from build123d import *

# Parameters (mm, degrees)
SM_BASE_FLANGE_1_DEPTH           = 3
SM_EDGE_FLANGE_1_STRIP_W         = 18
SM_EDGE_FLANGE_1_STRIP_H         = 3
SM_EDGE_FLANGE_1_STRIP_CUT_DEPTH = 130
SM_EDGE_FLANGE_1_DEPTH           = 130
SM_EDGE_FLANGE_2_DEPTH           = 52
SM_EDGE_FLANGE_5_DEPTH           = 52
CUT_EXTRUDE_2_REACH              = 158.911
SKETCH_48_R                      = 3.5
CUT_EXTRUDE_3_REACH              = 150.997
SKETCH_49_R                      = 3.5
CUT_EXTRUDE_4_REACH              = 150.997
SKETCH_51_R                      = 3.5
SM_EDGE_FLANGE_6_DEPTH           = 52
CUT_EXTRUDE_5_REACH              = 263.117
SKETCH_59_R                      = 3.5
SM_EDGE_FLANGE_8_DEPTH           = 130
CUT_EXTRUDE_6_REACH              = 229.141
SKETCH_68_R                      = 3.5
CUT_EXTRUDE_7_REACH              = 198.876
SKETCH_69_R                      = 3.5


# Sheet-metal steps are written as plain solids
with BuildPart() as part:
    # Sketch 2 → Базовая кромка1 (new body)
    with BuildSketch(Plane(origin=(0, 0, 0), x_dir=(1, 0, 0), z_dir=(0, 1, 0))):
        Polygon((45, 55), (130, 55), (130, 35), (45, 0), (0, 0), (0, 55), align=None)
    extrude(amount=-SM_BASE_FLANGE_1_DEPTH)

    # Ребро-кромка1 strip (across the edge) → Ребро-кромка1 strip cut (cut)
    with BuildSketch(Plane(origin=(0, -3, -55), x_dir=(0, 0, 1), z_dir=(1, 0, 0))):
        with Locations((-6, -1.5)):
            Rectangle(SM_EDGE_FLANGE_1_STRIP_W, SM_EDGE_FLANGE_1_STRIP_H)
    extrude(amount=SM_EDGE_FLANGE_1_STRIP_CUT_DEPTH, mode=Mode.SUBTRACT)

    # Ребро-кромка1 section (across the edge) → Ребро-кромка1 (add)
    with BuildSketch(Plane(origin=(0, -3, -55), x_dir=(0, 0, 1), z_dir=(1, 0, 0))):
        with BuildLine():
            Line((-3, 3), (-3, 20))
            Line((-3, 20), (0, 20))
            Line((0, 20), (0, 3))
            ThreePointArc((0, 3), (0.878679656, 0.878679656), (3, 0))
            Line((3, 0), (3, -3))
            ThreePointArc((3, -3), (-1.242640687, -1.242640687), (-3, 3))
        make_face()
    extrude(amount=SM_EDGE_FLANGE_1_DEPTH)

    # Ребро-кромка2 section (across the edge) → Ребро-кромка2 (add)
    with BuildSketch(Plane(origin=(-6, -3, 0), x_dir=(1, 0, 0), z_dir=(0, 0, -1))):
        with BuildLine():
            Line((-3, 3), (-3, 35))
            Line((-3, 35), (0, 35))
            Line((0, 35), (0, 3))
            ThreePointArc((0, 3), (0.878679656, 0.878679656), (3, 0))
            Line((3, 0), (6, 0))
            Line((6, 0), (6, -3))
            Line((6, -3), (3, -3))
            ThreePointArc((3, -3), (-1.242640687, -1.242640687), (-3, 3))
        make_face()
    extrude(amount=SM_EDGE_FLANGE_2_DEPTH)

    # Ребро-кромка5 section (across the edge) → Ребро-кромка5 (add)
    with BuildSketch(Plane(origin=(-9, -41, -52), x_dir=(0, 1, 0), z_dir=(0, 0, 1))):
        with BuildLine():
            Line((-3, 3), (-3, 38))
            Line((-3, 38), (0, 38))
            Line((0, 38), (0, 3))
            ThreePointArc((0, 3), (0.878679656, 0.878679656), (3, 0))
            Line((3, 0), (3, -3))
            ThreePointArc((3, -3), (-1.242640687, -1.242640687), (-3, 3))
        make_face()
    extrude(amount=SM_EDGE_FLANGE_5_DEPTH)

    # Эскиз48 → Вырез-Вытянуть2 (cut, up to next)
    with BuildSketch(Plane.ZY.offset(9), mode=Mode.PRIVATE) as cut_extrude_2_sk1:
        with Locations(Location((-41, -24, 0), (0, 0, 270))):
            Circle(SKETCH_48_R)
    cut_extrude_2_tool1 = extrude(cut_extrude_2_sk1.sketch, amount=-CUT_EXTRUDE_2_REACH, mode=Mode.PRIVATE) & part.part
    # Эскиз48 → Вырез-Вытянуть2 (cut, up to next)
    with BuildSketch(Plane.ZY.offset(9), mode=Mode.PRIVATE) as cut_extrude_2_sk2:
        with Locations(Location((-11, -24, 0), (0, 0, 270))):
            Circle(SKETCH_48_R)
    cut_extrude_2_tool2 = extrude(cut_extrude_2_sk2.sketch, amount=-CUT_EXTRUDE_2_REACH, mode=Mode.PRIVATE) & part.part
    add(cut_extrude_2_tool1.solids().sort_by_distance((-9, -24, -41))[0], mode=Mode.SUBTRACT)
    add(cut_extrude_2_tool2.solids().sort_by_distance((-9, -24, -11))[0], mode=Mode.SUBTRACT)

    # Эскиз49 → Вырез-Вытянуть3 (cut, up to next)
    with BuildSketch(Plane(origin=(0, 0, 0), x_dir=(1, 0, 0), z_dir=(0, 1, 0)), mode=Mode.PRIVATE) as cut_extrude_3_sk1:
        with Locations(Location((21, 12.448418776, 0), (0, 0, 270))):
            Circle(SKETCH_49_R)
    cut_extrude_3_tool1 = extrude(cut_extrude_3_sk1.sketch, amount=-CUT_EXTRUDE_3_REACH, mode=Mode.PRIVATE) & part.part
    # Эскиз49 → Вырез-Вытянуть3 (cut, up to next)
    with BuildSketch(Plane(origin=(0, 0, 0), x_dir=(1, 0, 0), z_dir=(0, 1, 0)), mode=Mode.PRIVATE) as cut_extrude_3_sk2:
        with Locations(Location((21, 38.45, 0), (0, 0, 270))):
            Circle(SKETCH_49_R)
    cut_extrude_3_tool2 = extrude(cut_extrude_3_sk2.sketch, amount=-CUT_EXTRUDE_3_REACH, mode=Mode.PRIVATE) & part.part
    # Эскиз49 → Вырез-Вытянуть3 (cut, up to next)
    with BuildSketch(Plane(origin=(0, 0, 0), x_dir=(1, 0, 0), z_dir=(0, 1, 0)), mode=Mode.PRIVATE) as cut_extrude_3_sk3:
        with Locations(Location((117, 38.45, 0), (0, 0, 270))):
            Circle(SKETCH_49_R)
    cut_extrude_3_tool3 = extrude(cut_extrude_3_sk3.sketch, amount=-CUT_EXTRUDE_3_REACH, mode=Mode.PRIVATE) & part.part
    # Эскиз49 → Вырез-Вытянуть3 (cut, up to next)
    with BuildSketch(Plane(origin=(0, 0, 0), x_dir=(1, 0, 0), z_dir=(0, 1, 0)), mode=Mode.PRIVATE) as cut_extrude_3_sk4:
        with Locations(Location((69, 38.45, 0), (0, 0, 270))):
            Circle(SKETCH_49_R)
    cut_extrude_3_tool4 = extrude(cut_extrude_3_sk4.sketch, amount=-CUT_EXTRUDE_3_REACH, mode=Mode.PRIVATE) & part.part
    add(cut_extrude_3_tool1.solids().sort_by_distance((21, 0, -12.448419))[0], mode=Mode.SUBTRACT)
    add(cut_extrude_3_tool2.solids().sort_by_distance((21, 0, -38.45))[0], mode=Mode.SUBTRACT)
    add(cut_extrude_3_tool3.solids().sort_by_distance((117, 0, -38.45))[0], mode=Mode.SUBTRACT)
    add(cut_extrude_3_tool4.solids().sort_by_distance((69, 0, -38.45))[0], mode=Mode.SUBTRACT)

    # Эскиз51 → Вырез-Вытянуть4 (cut, up to next)
    with BuildSketch(Plane(origin=(0, 0, -58), x_dir=(-1, 0, 0), z_dir=(0, 0, -1)), mode=Mode.PRIVATE) as cut_extrude_4_sk1:
        with Locations(Location((-117, -14.5, 0), (0, 0, 90))):
            Circle(SKETCH_51_R)
    cut_extrude_4_tool1 = extrude(cut_extrude_4_sk1.sketch, amount=-CUT_EXTRUDE_4_REACH, mode=Mode.PRIVATE) & part.part
    # Эскиз51 → Вырез-Вытянуть4 (cut, up to next)
    with BuildSketch(Plane(origin=(0, 0, -58), x_dir=(-1, 0, 0), z_dir=(0, 0, -1)), mode=Mode.PRIVATE) as cut_extrude_4_sk2:
        with Locations(Location((-69, -14.5, 0), (0, 0, 90))):
            Circle(SKETCH_51_R)
    cut_extrude_4_tool2 = extrude(cut_extrude_4_sk2.sketch, amount=-CUT_EXTRUDE_4_REACH, mode=Mode.PRIVATE) & part.part
    # Эскиз51 → Вырез-Вытянуть4 (cut, up to next)
    with BuildSketch(Plane(origin=(0, 0, -58), x_dir=(-1, 0, 0), z_dir=(0, 0, -1)), mode=Mode.PRIVATE) as cut_extrude_4_sk3:
        with Locations(Location((-21, -14.5, 0), (0, 0, 90))):
            Circle(SKETCH_51_R)
    cut_extrude_4_tool3 = extrude(cut_extrude_4_sk3.sketch, amount=-CUT_EXTRUDE_4_REACH, mode=Mode.PRIVATE) & part.part
    add(cut_extrude_4_tool1.solids().sort_by_distance((117, -14.5, -58))[0], mode=Mode.SUBTRACT)
    add(cut_extrude_4_tool2.solids().sort_by_distance((69, -14.5, -58))[0], mode=Mode.SUBTRACT)
    add(cut_extrude_4_tool3.solids().sort_by_distance((21, -14.5, -58))[0], mode=Mode.SUBTRACT)

    # Ребро-кромка6 section (across the edge) → Ребро-кромка6 (add)
    with BuildSketch(Plane(origin=(-50, -44, 0), x_dir=(1, 0, 0), z_dir=(0, 0, -1))):
        with BuildLine():
            Line((-3, 3), (-3, 133))
            Line((-3, 133), (0, 133))
            Line((0, 133), (0, 3))
            ThreePointArc((0, 3), (0.878679656, 0.878679656), (3, 0))
            Line((3, 0), (3, -3))
            ThreePointArc((3, -3), (-1.242640687, -1.242640687), (-3, 3))
        make_face()
    extrude(amount=SM_EDGE_FLANGE_6_DEPTH)

    # Эскиз59 → Вырез-Вытянуть5 (cut, up to next)
    with BuildSketch(Plane.ZY.offset(53), mode=Mode.PRIVATE) as cut_extrude_5_sk1:
        with Locations(Location((-7.981818004, -68, 0), (0, 0, 270))):
            Circle(SKETCH_59_R)
    cut_extrude_5_tool1 = extrude(cut_extrude_5_sk1.sketch, amount=-CUT_EXTRUDE_5_REACH, mode=Mode.PRIVATE) & part.part
    # Эскиз59 → Вырез-Вытянуть5 (cut, up to next)
    with BuildSketch(Plane.ZY.offset(53), mode=Mode.PRIVATE) as cut_extrude_5_sk2:
        with Locations(Location((-37.994919226, -68, 0), (0, 0, 270))):
            Circle(SKETCH_59_R)
    cut_extrude_5_tool2 = extrude(cut_extrude_5_sk2.sketch, amount=-CUT_EXTRUDE_5_REACH, mode=Mode.PRIVATE) & part.part
    # Эскиз59 → Вырез-Вытянуть5 (cut, up to next)
    with BuildSketch(Plane.ZY.offset(53), mode=Mode.PRIVATE) as cut_extrude_5_sk3:
        with Locations(Location((-37.994919226, -116, 0), (0, 0, 270))):
            Circle(SKETCH_59_R)
    cut_extrude_5_tool3 = extrude(cut_extrude_5_sk3.sketch, amount=-CUT_EXTRUDE_5_REACH, mode=Mode.PRIVATE) & part.part
    # Эскиз59 → Вырез-Вытянуть5 (cut, up to next)
    with BuildSketch(Plane.ZY.offset(53), mode=Mode.PRIVATE) as cut_extrude_5_sk4:
        with Locations(Location((-37.994919226, -164, 0), (0, 0, 270))):
            Circle(SKETCH_59_R)
    cut_extrude_5_tool4 = extrude(cut_extrude_5_sk4.sketch, amount=-CUT_EXTRUDE_5_REACH, mode=Mode.PRIVATE) & part.part
    # Эскиз59 → Вырез-Вытянуть5 (cut, up to next)
    with BuildSketch(Plane.ZY.offset(53), mode=Mode.PRIVATE) as cut_extrude_5_sk5:
        Polygon((0, -92), (-35, -177), (0, -177), align=None)
    cut_extrude_5_tool5 = extrude(cut_extrude_5_sk5.sketch, amount=-CUT_EXTRUDE_5_REACH, mode=Mode.PRIVATE) & part.part
    add(cut_extrude_5_tool1.solids().sort_by_distance((-53, -68, -7.981818))[0], mode=Mode.SUBTRACT)
    add(cut_extrude_5_tool2.solids().sort_by_distance((-53, -68, -37.994919))[0], mode=Mode.SUBTRACT)
    add(cut_extrude_5_tool3.solids().sort_by_distance((-53, -116, -37.994919))[0], mode=Mode.SUBTRACT)
    add(cut_extrude_5_tool4.solids().sort_by_distance((-53, -164, -37.994919))[0], mode=Mode.SUBTRACT)
    add(cut_extrude_5_tool5.solids().sort_by_distance((-53, -148.666667, -11.666667))[0], mode=Mode.SUBTRACT)

    # Ребро-кромка8 section (across the edge) → Ребро-кромка8 (add)
    with BuildSketch(Plane(origin=(-50, -177, -55), x_dir=(0, 0, 1), z_dir=(0, 1, 0))):
        with BuildLine():
            Line((-3, 3), (-3, 23))
            Line((-3, 23), (0, 23))
            Line((0, 23), (0, 3))
            ThreePointArc((0, 3), (0.878679656, 0.878679656), (3, 0))
            Line((3, 0), (3, -3))
            ThreePointArc((3, -3), (-1.242640687, -1.242640687), (-3, 3))
        make_face()
    extrude(amount=SM_EDGE_FLANGE_8_DEPTH)

    # Эскиз68 → Вырез-Вытянуть6 (cut, up to next)
    with BuildSketch(Plane(origin=(0, 0, -58), x_dir=(-1, 0, 0), z_dir=(0, 0, -1)), mode=Mode.PRIVATE) as cut_extrude_6_sk1:
        with Locations((35.5, -68)):
            Circle(SKETCH_68_R)
    cut_extrude_6_tool1 = extrude(cut_extrude_6_sk1.sketch, amount=-CUT_EXTRUDE_6_REACH, mode=Mode.PRIVATE) & part.part
    # Эскиз68 → Вырез-Вытянуть6 (cut, up to next)
    with BuildSketch(Plane(origin=(0, 0, -58), x_dir=(-1, 0, 0), z_dir=(0, 0, -1)), mode=Mode.PRIVATE) as cut_extrude_6_sk2:
        with Locations((35.5, -116)):
            Circle(SKETCH_68_R)
    cut_extrude_6_tool2 = extrude(cut_extrude_6_sk2.sketch, amount=-CUT_EXTRUDE_6_REACH, mode=Mode.PRIVATE) & part.part
    # Эскиз68 → Вырез-Вытянуть6 (cut, up to next)
    with BuildSketch(Plane(origin=(0, 0, -58), x_dir=(-1, 0, 0), z_dir=(0, 0, -1)), mode=Mode.PRIVATE) as cut_extrude_6_sk3:
        with Locations((35.5, -164)):
            Circle(SKETCH_68_R)
    cut_extrude_6_tool3 = extrude(cut_extrude_6_sk3.sketch, amount=-CUT_EXTRUDE_6_REACH, mode=Mode.PRIVATE) & part.part
    add(cut_extrude_6_tool1.solids().sort_by_distance((-35.5, -68, -58))[0], mode=Mode.SUBTRACT)
    add(cut_extrude_6_tool2.solids().sort_by_distance((-35.5, -116, -58))[0], mode=Mode.SUBTRACT)
    add(cut_extrude_6_tool3.solids().sort_by_distance((-35.5, -164, -58))[0], mode=Mode.SUBTRACT)

    # Эскиз69 → Вырез-Вытянуть7 (cut, up to next)
    with BuildSketch(Plane(origin=(0, -41, 0), x_dir=(1, 0, 0), z_dir=(0, 1, 0)), mode=Mode.PRIVATE) as cut_extrude_7_sk1:
        with Locations(Location((-30, 42.45, 0), (0, 0, 270))):
            Circle(SKETCH_69_R)
    cut_extrude_7_tool1 = extrude(cut_extrude_7_sk1.sketch, amount=-CUT_EXTRUDE_7_REACH, mode=Mode.PRIVATE) & part.part
    # Эскиз69 → Вырез-Вытянуть7 (cut, up to next)
    with BuildSketch(Plane(origin=(0, -41, 0), x_dir=(1, 0, 0), z_dir=(0, 1, 0)), mode=Mode.PRIVATE) as cut_extrude_7_sk2:
        with Locations(Location((-30, 12.45, 0), (0, 0, 270))):
            Circle(SKETCH_69_R)
    cut_extrude_7_tool2 = extrude(cut_extrude_7_sk2.sketch, amount=-CUT_EXTRUDE_7_REACH, mode=Mode.PRIVATE) & part.part
    add(cut_extrude_7_tool1.solids().sort_by_distance((-30, -41, -42.45))[0], mode=Mode.SUBTRACT)
    add(cut_extrude_7_tool2.solids().sort_by_distance((-30, -41, -12.45))[0], mode=Mode.SUBTRACT)


solid = part.part
Work out the finished part from the listing and answer in its coordinate system (mm). A direction names the side the tool comes from. Coordinates: 2 decimals unless noted, no trailing zeros. Order: outer loops, then holes, each group sorted by start corner. A loop starts at its lowest first (then second) coordinate and runs counter-clockwise, first axis right, second up. Notation, with made-up numbers: (39.5, 74.25) - (53.5, 74.25) arc R34 cw to (53.5, 110.25) - close; hole circle Ø10 at (74, -21). An arc over 180 degrees is marked (long way). Put each result on its own line as item: value. Start each with the question number.
1) For a pull along X with two mould halves and no side action, classify faces 1 (the cylindrical face through (-7.521, -27.233, -12.341)), 2 (the cylindrical face through (-32, -68, -57)), 3 (the flat face through (-50, -98, -31)) as released by +X, released by -X, zero draft, split by the parting line, or undercut.
2) Flat-ended cylindrical pins translate along their axes: pin 1 (8 mm diameter, centred on x = -30, z = -12.45, fed in from -Y); pin 2 (1.5 mm diameter, centred on x = 67.5, z = -24.5, fed in from -Y); pin 3 (13.5 mm diameter, centred on x = 74, y = -17, fed in from +Z); pin 4 (6.5 mm diameter, centred on x = 69, y = -14.5, fed in from +Z). Find the tip coordinate at first contact, or state that the pin passes through.
3) Find section A-A (y = -68). Give the vertices of the cut face in (x, z), plus the area to 3 significant figures.
4) Find section D-D (z = -30). Give the vertices of the cut face in (x, y).
5) Find section C-C (x = 69). Give the vertices of the cut face in (y, z), plus the area to 3 significant figures.
6) Find the intervals of material crossed by line 1 (X direction, y = -2.15, z = -38.45); line 2 (X direction, y = -115.5, z = -52); line 3 (Y direction, x = 2, z = -37), in increasing order. Write a range as from..to.
7) Find section B-B (x = 21). Give the vertices of the cut face in (y, z).
8) For faces 4 (the flat face through (-6, -22, -26)), 5 (the flat face through (48, -3, -31)), 6 (the cylindrical face through (-7.52, -23.54, -37.53)), 7 (the flat face through (-30, -41, -26)), determine the directions among +Z, -Z, +X, -X, +Y, -Y from which every point of the face is accessible in a straight line to the end or side of a thin tool.
Results list:
1. face 1: zero draft
1. face 2: undercut
1. face 3: released by +X
2. pin 1: stops at y = -44
2. pin 2: stops at y = -3
2. pin 3: stops at z = -55
2. pin 4: passes through
3. outline: (-53, -52) arc R6 ccw to (-47, -58) - (-39, -58) - (-39, -55) - (-47, -55) arc R3 cw to (-50, -52) - (-50, -41.49) - (-53, -41.49) - close; (-53, -34.49) - (-50, -34.49) - (-50, -11.48) - (-53, -11.48) - close; (-53, -4.48) - (-50, -4.48) - (-50, 0) - (-53, 0) - close; (-32, -58) - (-27, -58) - (-27, -55) - (-32, -55) - close
3. area: 174 mm^2
4. outline: (-53, -164.86) - (-50, -164.86) - (-50, -47) arc R3 cw to (-47, -44) - (-12, -44) arc R6 ccw to (-6, -38) - (-6, -6) arc R3 cw to (-3, -3) - (117.86, -3) - (117.86, 0) - (-3, 0) arc R6 ccw to (-9, -6) - (-9, -38) arc R3 cw to (-12, -41) - (-47, -41) arc R6 ccw to (-53, -47) - close
5. outline: (-23, -58) - (-18, -58) - (-18, -55) - (-23, -55) - close; (-11, -58) - (-6, -58) arc R6 ccw to (0, -52) - (0, -41.95) - (-3, -41.95) - (-3, -52) arc R3 cw to (-6, -55) - (-11, -55) - close; (-3, -34.95) - (0, -34.95) - (0, -9.88) - (-3, -9.88) - close
5. area: 157 mm^2
6. line 1: x = -7.6..17.5, 24.5..65.5, 72.5..113.5, 120.5..130
6. line 2: x = -53..-50
6. line 3: y = -3..0
7. outline: (-23, -58) - (-18, -58) - (-18, -55) - (-23, -55) - close; (-11, -58) - (-6, -58) arc R6 ccw to (0, -52) - (0, -41.95) - (-3, -41.95) - (-3, -52) arc R3 cw to (-6, -55) - (-11, -55) - close; (-3, -34.95) - (0, -34.95) - (0, -15.95) - (-3, -15.95) - close; (-3, -8.95) - (0, -8.95) - (0, 0) - (-3, 0) - close
8. face 4: +Z, -Z, +X, -Y
8. face 5: +Z, +X, -Y
8. face 6: +X, -X
8. face 7: +Z, -Z, -X, +Y
